Geometry check sheet. Reference: the model listing, model coordinates, mm. A direction names the side the tool comes from. Coordinates: 2 decimals unless noted, no trailing zeros. Write each loop counter-clockwise with the first axis right and the second up, starting at its lowest first coordinate (ties: lowest second). Pieces come first, ordered by that corner, then holes. Notation, with made-up numbers: (38, -19.75) -> (83, -19.75) arc R21 cw to (83, 1.25) -> close; hole circle Ø6 at (80, 23.5). An arc over 180 degrees is marked (long way). Answer in a Markdown table with one row per item. Add a question column.
1. Scan lines: L1, parallel to Y at x = 21.75, z = 5.25; L2, parallel to Z at x = 21.9, y = -12.25. Record each from-to range of solid material in increasing order. Write a range as from..to.
2. Cross-section at B-B on z = 5.5. Record the cut outline in (x, y), and give its area (3 significant figures).
3. Mould release check, pull along Z, two halves, no side actions. Record for faces 1 (the flat face through (22, -10, 7)), 2 (the flat face through (22, -10, -2)), 3 (the flat face through (22, -11.5, -1)): pulls with the +Z half, pulls with the -Z half, needs draft (parallel to the pull), parting line crosses it, or undercut.
4. Set-up check for faces 4 (the flat face through (22, -9, 2)), 5 (the flat face through (22, -13, 0)), 6 (the flat face through (22, -13, 5)): record each of +Z, -Z, +X, -X, +Y, -Y from which the full face is reachable in a straight line by a thin tool's end or side.
5. Cross-section at C-C on y = -12.2. Record the cut outline in (x, z), and give its area (3 significant figures).
6. Cross-section at A-A on x = 21.1. Record the cut outline in (y, z).
7. Depth check by flat-ended pin: P1, Ø1, axis at x = 22, z = -1, coming from the -Y side. Enter the tip coordinate at first touch or a pass-through.
Autodesk Inventor part; units mm, degrees
ref_plane "YZ Plane" through (0, 0, 0) normal (1, 0, 0) x (0, 1, 0)
ref_plane "XZ Plane" through (0, 0, 0) normal (0, 1, 0) x (-1, 0, 0)
ref_plane "XY Plane" through (0, 0, 0) normal (0, 0, 1) x (1, 0, 0)
ref_plane "Work Plane1" through (2.9206, -11.5, 0) normal (0, 1, 0) x (1, 0, 0)
sketch "Sketch1" plane through (2.9206, -11.5, 0) normal (0, 1, 0) x (1, 0, 0)
  line L0 (0, 0) -> (30, 0)
  line L1 (30, 0) -> (30, 2)
  line L2 (20, 2) -> (30, 2)
  line L3 (20, 2) -> (20, 4)
  line L4 (18, 4) -> (20, 4)
  line L5 (18, 2) -> (18, 4)
  line L6 (15, 2) -> (18, 2)
  line L7 (15, 2) -> (15, 4)
  line L8 (13, 4) -> (15, 4)
  line L9 (13, 2) -> (13, 4)
  line L10 (0, 2) -> (13, 2)
  line L11 (0, 0) -> (0, 2)
  line L12 (18, 2) -> (18, 0)
  line L13 (18, 2) -> (20, 2)
  line L14 (20, 2) -> (20, 0)
  line L15 (18, 0) -> (20, 0)
  line L16 (18, 0) -> (18, -5)
  line L17 (18, -5) -> (20, -5)
  line L18 (20, -5) -> (20, 0)
  line L19 (18, -5) -> (18, -7)
  line L20 (18, -7) -> (20, -7)
  line L21 (20, -7) -> (20, -5)
  point P0 (-2.9206, 0)
  dimension "d7" = 5
  dimension "d8" = 2
ref_plane "Work Plane2" through (2.9206, -11.5, 0) normal (0, -1, 0) x (1, 0, 0)
extrude "Extrusion3" add sketch "Sketch1" along normal blind 2.5 contours L12 L13 L14 L0 | L0 L18 L17 L16 | L17 L21 L20 L19
sketch "Sketch3" plane through (2.9206, -11.5, 0) normal (0, -1, 0) x (1, 0, 0)
  line L0 (20, 7) -> (20, -2)
  line L1 (2, 0) -> (28, 0)
  line L2 (20, 0) -> (20, 5)
  line L3 (20, 7) -> (20, -2)
  line L4 (20, 5) -> (18, 5)
  line L5 (18, -2) -> (18, 7)
  line L6 (18, 5) -> (18, 0)
  line L7 (20, 0) -> (18, 0)
  point P0 (-2.9206, 0)
  dimension "d11" = 5
extrude "Extrusion4" add sketch "Sketch3" along normal blind 2.5
properties part number "spacer_"
Results found:
| question | item | result |
|---|---|---|
| 1 | L1 | y = -11.5..-9 |
| 1 | L2 | z = 0..5 |
| 2 | outline | (20.92, -11.5) -> (22.92, -11.5) -> (22.92, -9) -> (20.92, -9) -> close |
| 2 | area | 5.00 mm^2 |
| 3 | face 1 | pulls with the +Z half |
| 3 | face 2 | pulls with the -Z half |
| 3 | face 3 | needs draft |
| 4 | face 4 | +Z, -Z, +X, -X, +Y |
| 4 | face 5 | -Z, +X, -X, -Y |
| 4 | face 6 | +Z, +X, -X, -Y |
| 5 | outline | (20.92, 0) -> (22.92, 0) -> (22.92, 5) -> (20.92, 5) -> close |
| 5 | area | 10.0 mm^2 |
| 6 | outline | (-14, 0) -> (-11.5, 0) -> (-11.5, -2) -> (-9, -2) -> (-9, 7) -> (-11.5, 7) -> (-11.5, 5) -> (-14, 5) -> close |
| 7 | P1 | stops at y = -11.5 |
